Geometry check sheet. Reference: the model listing, model coordinates, mm. A direction names the side the tool comes from. Give positions to 0.01 mm unless a question says otherwise; leave off trailing zeros. Write each loop counter-clockwise with the first axis right and the second up, starting at its lowest first coordinate (ties: lowest second). Pieces come first, ordered by that corner, then holes. Notation, with made-up numbers: (7, 33.5) -> (25, 33.5) arc R36 ccw to (25, 70.5) -> close; hole circle Ø6 at (31, 20.5). An arc over 180 degrees is marked (long way). Write item = value, one per line. Start each with the question number.
1. Cross-section at B-B, the plane z = -2.5. Record the cut outline in (x, y) (3 decimals), plus the area to 3 significant figures.
2. Cross-section at D-D, the plane x = 1.5. State how many separate pieces and enclosed holes the cut face has, plus the area to 3 significant figures.
3. Mould release check, pull along Z, two halves, no side actions. Record for faces 6 (the flat face through (2, 19, -33.25)), 7 (the flat face through (2, 30, -6.35)), 8 (the flat face through (2, 31.75, 7)): pulls with the +Z half, pulls with the -Z half, needs draft (parallel to the pull), parting line crosses it, or undercut.
4. Thickness scan on line 1 along Y through (x, z) = (3.05, -34.5) (3 decimals); line 2 along Z through (x, y) = (0.6, 25); line 3 along Z through (x, y) = (1.6, 21). Record the ranges inside material, lowest first.
5. Depth check by flat-ended pin: P1, Ø1, axis at x = 1.5, z = 34, coming from the -Y side (3 decimals); P2, Ø1.5, axis at x = 1.5, z = -32, coming from the +Y side (3 decimals); P3, Ø1, axis at x = 1.5, z = -17, coming from the +Y side (3 decimals). Enter the tip coordinate at first touch or a pass-through.
6. Cross-section at C-C, the plane z = 35.5. Record the cut outline in (x, y) (3 decimals), plus the area to 3 significant figures.
7. Set-up check for faces 1 (the flat face through (2, -28.575, -18)), 2 (the flat face through (2, -28.575, 39)), 3 (the flat face through (2, 19, -30.25)), 4 (the flat face through (2, -21, -34.55)), 5 (the flat face through (2, -19, -30.25)): record each of +Z, -Z, +X, -X, +Y, -Y from which the full face is reachable in a straight line by a thin tool's end or side.
8. Cross-section at A-A, the plane y = 25.5. Record the cut outline in (x, z) (3 decimals), plus the area to 3 significant figures.
```python
from build123d import *

# Parameters (mm, degrees)
SKETCH1_W           = 88.9
SKETCH1_H           = 63.5
BOSS_EXTRUDE1_DEPTH = 3.175
SKETCH2_W           = 38.1
SKETCH2_H           = 3.175
CUT_EXTRUDE1_DEPTH  = 55.716959208
CUT_EXTRUDE2_DEPTH  = 55.716959208
SKETCH4_R           = 6.35
SKETCH4_R_2         = 1.27
CUT_EXTRUDE3_DEPTH  = 55.716959208


with BuildPart() as part:
    # Sketch1 → Boss-Extrude1 (new body)
    with BuildSketch(Plane(origin=(0, 0, 0), x_dir=(0, 0, -1), z_dir=(1, 0, 0))):
        Rectangle(SKETCH1_W, SKETCH1_H)
    extrude(amount=BOSS_EXTRUDE1_DEPTH)

    # Sketch2 → Cut-Extrude1 (cut, through all)
    with BuildSketch(Plane(origin=(3.175, 0, 0), x_dir=(0, 0, -1), z_dir=(1, 0, 0))):
        with Locations((25.4, -30.1625)):
            Rectangle(SKETCH2_W, SKETCH2_H)
        Polygon((-19.05, 28.575), (-44.45, 28.575), (-44.45, 31.75), (-41.275, 31.75), (-19.05, 31.75), align=None)
        Polygon((-44.45, -31.75), (-41.275, -31.75), (-19.05, -31.75), (-19.05, -28.575), (-44.45, -28.575), align=None)
        with Locations((25.4, 30.1625)):
            Rectangle(SKETCH2_W, SKETCH2_H)
    extrude(amount=-CUT_EXTRUDE1_DEPTH, mode=Mode.SUBTRACT)

    # Sketch3 → Cut-Extrude2 (cut, through all)
    with BuildSketch(Plane(origin=(3.175, 0, 0), x_dir=(0, 0, -1), z_dir=(1, 0, 0))):
        Polygon((-30.25, -17.575), (-30.25, -20.125), (-28.95, -20.125), (-28.95, -22.025), (-30.25, -22.025), (-30.25, -28.575), (-33.25, -28.575), (-33.25, -22.025), (-34.55, -22.025), (-34.55, -20.125), (-33.25, -20.125), (-33.25, -17.575), align=None)
        Polygon((33.25, -17.575), (33.25, -20.125), (34.55, -20.125), (34.55, -22.025), (33.25, -22.025), (33.25, -28.575), (30.25, -28.575), (30.25, -22.025), (28.95, -22.025), (28.95, -20.125), (30.25, -20.125), (30.25, -17.575), align=None)
        Polygon((33.25, 20.125), (34.55, 20.125), (34.55, 22.025), (33.25, 22.025), (33.25, 28.575), (30.25, 28.575), (30.25, 22.025), (28.95, 22.025), (28.95, 20.125), (30.25, 20.125), (30.25, 17.575), (33.25, 17.575), align=None)
        Polygon((-30.25, 20.125), (-28.95, 20.125), (-28.95, 22.025), (-30.25, 22.025), (-30.25, 28.575), (-33.25, 28.575), (-33.25, 22.025), (-34.55, 22.025), (-34.55, 20.125), (-33.25, 20.125), (-33.25, 17.575), (-30.25, 17.575), align=None)
    extrude(amount=-CUT_EXTRUDE2_DEPTH, mode=Mode.SUBTRACT)

    # Sketch4 → Cut-Extrude3 (cut, through all)
    with BuildSketch(Plane(origin=(3.175, 0, 0), x_dir=(0, 0, -1), z_dir=(1, 0, 0))):
        with Locations((1.09372, 14.225)):
            Circle(SKETCH4_R)
        with Locations((-7.198382525, 5.625)):
            Circle(SKETCH4_R_2)
        with Locations((-7.198382525, 22.825)):
            Circle(SKETCH4_R_2)
    extrude(amount=-CUT_EXTRUDE3_DEPTH, mode=Mode.SUBTRACT)


solid = part.part
```
Answers:
q1.outline = (0, -31.75) -> (3.175, -31.75) -> (3.175, 8.033) -> (0, 8.033) -> close; (0, 20.417) -> (3.175, 20.417) -> (3.175, 31.75) -> (0, 31.75) -> close
q1.area = 162 mm^2
q2.separate_pieces = 1
q2.enclosed_holes = 3
q2.area = 4,950 mm^2
q3.face_6 = undercut
q3.face_7 = pulls with the -Z half
q3.face_8 = needs draft
q4.line_1 = -28.575 to -22.025, -20.125 to 20.125, 22.025 to 28.575
q4.line_2 = -44.45 to -33.25, -30.25 to 30.25, 33.25 to 44.45
q4.line_3 = -44.45 to -34.55, -28.95 to 28.95, 34.55 to 44.45
q5.P1 = -28.575
q5.P2 = 17.575
q5.P3 = 28.575
q6.outline = (0, -28.575) -> (3.175, -28.575) -> (3.175, 28.575) -> (0, 28.575) -> close
q6.area = 181 mm^2
q7.face_1 = -Z, +X, -X, -Y
q7.face_2 = +Z, +X, -X, -Y
q7.face_3 = +X, -X, +Y
q7.face_4 = +X, -X
q7.face_5 = +X, -X, -Y
q8.outline = (0, -44.45) -> (3.175, -44.45) -> (3.175, -33.25) -> (0, -33.25) -> close; (0, -30.25) -> (3.175, -30.25) -> (3.175, 30.25) -> (0, 30.25) -> close; (0, 33.25) -> (3.175, 33.25) -> (3.175, 44.45) -> (0, 44.45) -> close
q8.area = 263 mm^2
